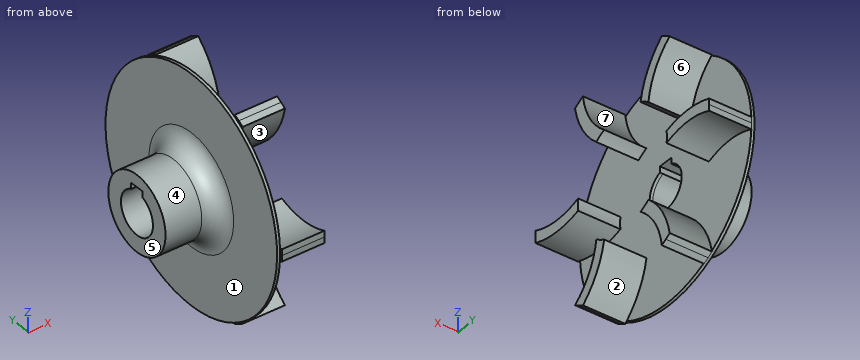
```python
from build123d import *

# Parameters (mm, degrees)
SKETCH3_R           = 37.5
BOSS_EXTRUDE1_DEPTH = 1
SKETCH4_R           = 12.5
BOSS_EXTRUDE2_DEPTH = 18
FILLET1_R           = 6
BOSS_EXTRUDE4_START = 14
BOSS_EXTRUDE4_DEPTH = 14
CIRPATTERN1_COUNT   = 6
CUT_EXTRUDE1_START  = -14
CUT_EXTRUDE1_DEPTH  = 14


with BuildPart() as part:
    # Sketch3 → Boss-Extrude1 (new body)
    with BuildSketch(Plane.YZ):
        with Locations(Location((0, 0, 0), (0, 0, 270))):
            Circle(SKETCH3_R)
    extrude(amount=-BOSS_EXTRUDE1_DEPTH)

    # Sketch4 → Boss-Extrude2 (add)
    with BuildSketch(Plane(origin=(-1, 0, 0), x_dir=(0, -1, 0), z_dir=(-1, 0, 0))):
        with Locations(Location((0, 0, 0), (0, 0, 270))):
            Circle(SKETCH4_R)
        with BuildLine():
            Line((-2.5, 8.538348415), (2.5, 8.538348415))
            Line((2.5, 8.538348415), (2.5, 6.538348415))
            ThreePointArc((2.5, 6.538348415), (0, -7), (-2.5, 6.538348415))
            Line((-2.5, 6.538348415), (-2.5, 8.538348415))
        make_face(mode=Mode.SUBTRACT)
    extrude(amount=BOSS_EXTRUDE2_DEPTH)

    # Fillet1
    fillet1_edges = [part.edges().sort_by_distance(p)[0] for p in [
        (-1, 0, 12.5),
    ]]
    fillet(fillet1_edges, radius=FILLET1_R)

    # Sketch7 → Boss-Extrude4 (add)
    with BuildSketch(Plane.YZ.offset(BOSS_EXTRUDE4_START)):
        with BuildLine():
            ThreePointArc((37.447145172, -1.990306119), (37.486783964, -0.995503903), (37.5, 0))
            ThreePointArc((37.5, 0), (37.486783964, 0.995503903), (37.447145172, 1.990306119))
            ThreePointArc((37.447145172, 1.990306119), (28.171306197, 3.571396011), (18.895467222, 1.990306119))
            ThreePointArc((18.895467222, 1.990306119), (19, 0), (18.895467222, -1.990306119))
            ThreePointArc((18.895467222, -1.990306119), (28.171306197, -0.148603989), (37.447145172, -1.990306119))
        make_face()
    boss_extrude4 = extrude(amount=-BOSS_EXTRUDE4_DEPTH)

    # CirPattern1: Boss-Extrude4 ×6 about axis
    cirpattern1_axis = Axis((0, -0.457216439, -0.018479017), (1, 0, 0))
    for i in range(1, CIRPATTERN1_COUNT):
        add(boss_extrude4.rotate(cirpattern1_axis, i * 360 / CIRPATTERN1_COUNT))

    # Sketch4<2> → Cut-Extrude1 (cut)
    with BuildSketch(Plane(origin=(-1, 0, 0), x_dir=(0, -1, 0), z_dir=(-1, 0, 0)).offset(CUT_EXTRUDE1_START)):
        with BuildLine():
            Line((-2.5, 8.538348415), (-2.5, 6.538348415))
            ThreePointArc((-2.5, 6.538348415), (0, -7), (2.5, 6.538348415))
            Line((2.5, 6.538348415), (2.5, 8.538348415))
            Line((2.5, 8.538348415), (-2.5, 8.538348415))
        make_face()
    extrude(amount=CUT_EXTRUDE1_DEPTH, mode=Mode.SUBTRACT)


solid = part.part
```
Can you work these out from the model? Positions are in its coordinate system, mm. Face numbers are marked on the shaded views. A direction names the side the tool comes from. Round coordinates to 2 decimals unless told otherwise and drop trailing zeros. Loops run counter-clockwise (first coordinate to the right, second up) from the corner with the lowest first, then second, coordinate; pieces in that order, holes last. Notation, with made-up numbers: M -5,-9 L 53,-9 A8 ccw 53,0 Z; hole C 5,-15.75 d7. An arc over 180 degrees is marked long. Answer in a Markdown table with one row per item.
1. If we section it at D-D, the plane x = -9: Please give me the cut outline in (y, z).
Established:
| item | result |
|---|---|
| outline | C 0,0 d25; hole M -2.5,6.54 A7 ccw long 2.5,6.54 L 2.5,8.54 L -2.5,8.54 Z |
2. Thinking about a two-plate mould opening in Y: for the marked faces 1, 2 and 3, which applies, pulls with the +Y half, pulls with the -Y half, needs draft (parallel to the pull), parting line crosses it, or undercut?
Established:
| item | result |
|---|---|
| face 1 | needs draft |
| face 2 | undercut |
| face 3 | pulls with the -Y half |
3. Please list where these lines run through material, in increasing order: line 1 (X direction, y = -26, z = -9.5); line 2 (Y direction, x = -0.6, z = 0); line 3 (Y direction, x = -14, z = 0). Write a range as from..to.
Established:
| item | result |
|---|---|
| line 1 | -1..0 |
| line 2 | -37.5..-7, 7..37.5 |
| line 3 | -12.5..-7, 7..12.5 |
4. If we section it at A-A, the plane y = 0: Please give me the cut outline in (x, z).
Established:
| item | result |
|---|---|
| outline | M -19,-12.5 L -7,-12.5 A6 cw -1,-18.5 L -1,-37.5 L 0,-37.5 L 0,-7 L -19,-7 Z; M -19,8.54 L 0,8.54 L 0,37.5 L -1,37.5 L -1,18.5 A6 cw -7,12.5 L -19,12.5 Z |
5. On a 3-axis mill with a long thin cutter (end or side, diameter ignored), from which of +Z, -Z, +X, -X, +Y, -Y can I reach the whole of each face in a straight line? I mean the marked faces 4, 5, 6 and 7. Say none if no direction works.
Established:
| item | result |
|---|---|
| face 4 | -X |
| face 5 | +Z, -Z, -X, +Y, -Y |
| face 6 | +X, +Y |
| face 7 | +Z, +X |
6. If we section it at B-B, the plane x = 1.5: Please give me the cut outline in (y, z), plus the area to 3 significant figures.
Established:
| item | result |
|---|---|
| outline | M -38.36,-2.03 A28 ccw -19.81,-2.03 A19 cw -19.81,1.95 A24.28 cw -38.36,1.95 A37.5 ccw Z; M -21.15,31.8 A28 ccw -11.87,15.74 A19 cw -8.43,17.73 A24.28 cw -17.7,33.79 A37.5 ccw Z; M -21.12,-31.86 A37.5 ccw -17.67,-33.85 A28 ccw -8.39,-17.78 A19 cw -11.84,-15.79 A24.28 cw Z; M 7.48,17.75 A19 cw 10.93,15.76 A24.28 cw 20.2,31.82 A37.5 ccw 16.76,33.81 A28 ccw Z; M 7.51,-17.76 A24.28 cw 16.79,-33.83 A37.5 ccw 20.23,-31.84 A28 ccw 10.96,-15.77 A19 cw Z; M 18.9,-1.99 A24.28 cw 37.45,-1.99 A37.5 ccw 37.45,1.99 A28 ccw 18.9,1.99 A19 cw Z |
| area | 423 mm² |
7. I'm going to push flat-ended pins straight in: pin 1 Ø3 at (y, z) = (1.5, 23) entering from -X; pin 2 Ø11 at (y, z) = (0, 0) entering from +X; pin 3 Ø1.5 at (x, y) = (-5.5, 0) entering from -Z; pin 4 Ø1 at (x, z) = (-12, 8) entering from -Y. Where does each tip first touch, or does it pass through?
Established:
| item | result |
|---|---|
| pin 1 | x = -1 |
| pin 2 | through |
| pin 3 | z = -12.94 |
| pin 4 | y = -10 |
8. If we section it at C-C, the plane z = 24.5: Please give me the cut outline in (x, y).
Established:
| item | result |
|---|---|
| outline | M -1,-28.39 L 0,-28.39 L 0,-18.7 L 14,-18.7 L 14,-14.46 L 0,-14.46 L 0,9.67 L 14,9.67 L 14,13.85 L 0,13.85 L 0,28.39 L -1,28.39 Z |
